Geometry: see drawing. Coordinates: mm, zero at the bounding-box minimum. A direction names the side the tool comes from. Give positions to 0.01 mm unless a question says otherwise; leave off trailing zeros. Loops run counter-clockwise (first coordinate to the right, second up) from the corner with the lowest first, then second, coordinate; pieces in that order, holes last. Notation, with made-up numbers: M -35.75,80 L -21.75,80 A10 ccw -21.75,85 Z; hole C -32,19 d11. An arc over 180 degrees is marked long. Return JSON: item names as keys, results as strings. Group by question number.
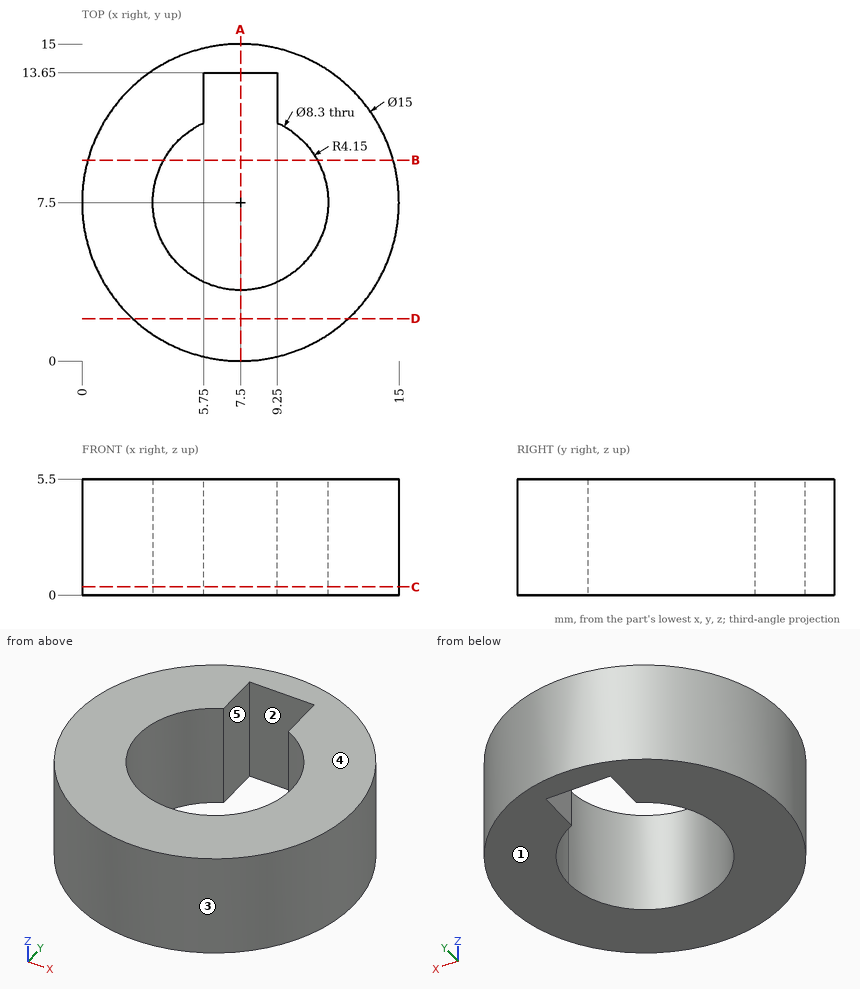
Item 1: First-contact query: pin 1 Ø1.9 at (y, z) = (12, 2) entering from +X; pin 2 Ø1 at (y, z) = (11, 4) entering from -X; pin 3 Ø1 at (x, y) = (10, 2.5) entering from -Z; pin 4 Ø1.5 at (y, z) = (9, 3.5) entering from -X. Flat tips, straight axial feed; report the tip coordinate or a pass-through.
Item 2: Pull-direction query (X, two-part tool) for the marked faces 3, 4 and 5; classes: pulls with the +X half, pulls with the -X half, needs draft (parallel to the pull), parting line crosses it, or undercut.
Item 3: Section D-D, the plane y = 2. Return loops of the section in (x, z).
Item 4: Section B-B, the plane y = 9.5. Return loops of the section in (x, z), then the cut area to 3 significant figures.
Item 5: Reachability of the marked faces 1 and 2 from +Z, -Z, +X, -X, +Y, -Y: full face, straight path, thin tool, end or side. Return the list, or none.
Item 6: Section C-C, the plane z = 0.4. Return loops of the section in (x, y), then the cut area to 3 significant figures.
Item 7: Material intervals for line 1 (Y direction, x = 7.5, z = 3.45); line 2 (X direction, y = 12, z = 0.85); line 3 (X direction, y = 11.5, z = 0.75), sorted ascending. Write a range as from..to.
Item 8: Section A-A, the plane x = 7.5. Return loops of the section in (y, z).
Answer below:
{
 "1": {"pin 1": "x = 14.11", "pin 2": "x = 0.63", "pin 3": "z = 0", "pin 4": "x = 0.04"},
 "2": {"face 3": "parting line crosses it", "face 4": "needs draft", "face 5": "undercut"},
 "3": {"outline": "M 2.4,0 L 12.6,0 L 12.6,5.5 L 2.4,5.5 Z"},
 "4": {"outline": "M 0.27,0 L 3.86,0 L 3.86,5.5 L 0.27,5.5 Z; M 11.14,0 L 14.73,0 L 14.73,5.5 L 11.14,5.5 Z", "area": "39.5 mm^2"},
 "5": {"face 1": "-Z, +X, -X, +Y, -Y", "face 2": "+Z, -Z"},
 "6": {"outline": "C 7.5,7.5 d15; hole M 5.75,11.26 A4.15 ccw long 9.25,11.26 L 9.25,13.65 L 5.75,13.65 Z", "area": "115 mm^2"},
 "7": {"line 1": "0..3.35, 13.65..15", "line 2": "1.5..5.75, 9.25..13.5", "line 3": "1.16..5.75, 9.25..13.84"},
 "8": {"outline": "M 0,0 L 3.35,0 L 3.35,5.5 L 0,5.5 Z; M 13.65,0 L 15,0 L 15,5.5 L 13.65,5.5 Z"}
}
